```python
from build123d import *

# Parameters (mm, degrees)
SKETCH1_R                    = 77.5
SKETCH1_R_2                  = 56
BOSS_EXTRUDE1_DEPTH          = 5
SKETCH2_R                    = 2.75
CUT_EXTRUDE2_DEPTH           = 110.715541287
CHAMFER1_SIZE                = 0.5
CIRPATTERN1_COUNT            = 6
CHAMFER1_OF_CIRPATTERN1_SIZE = 0.5
CHAMFER2_SIZE                = 1


with BuildPart() as part:
    # Sketch1 → Boss-Extrude1 (new body)
    with BuildSketch(Plane(origin=(0, 0, 0), x_dir=(1, 0, 0), z_dir=(0, 1, 0))):
        with Locations(Location((0, 0, 0), (0, 0, 270))):
            Circle(SKETCH1_R)
        with Locations(Location((0, 0, 0), (0, 0, 270))):
            Circle(SKETCH1_R_2, mode=Mode.SUBTRACT)
    extrude(amount=BOSS_EXTRUDE1_DEPTH)

    # Sketch2 → Cut-Extrude2 (cut, through all)
    with BuildSketch(Plane(origin=(0, 5, 0), x_dir=(1, 0, 0), z_dir=(0, 1, 0))):
        with Locations(Location((0, 70.25, 0), (0, 0, 270))):
            Circle(SKETCH2_R)
    cut_extrude2 = extrude(amount=-CUT_EXTRUDE2_DEPTH, mode=Mode.SUBTRACT)

    # Chamfer1
    chamfer1_edges = [part.edges().sort_by_distance(p)[0] for p in [
        (0, 0, -73),
        (0, 5, -73),
    ]]
    chamfer(chamfer1_edges, length=CHAMFER1_SIZE)

    # CirPattern1: Cut-Extrude2 ×6 about axis
    cirpattern1_axis = Axis((0, 0, 0), (0, 1, 0))
    for i in range(1, CIRPATTERN1_COUNT):
        add(cut_extrude2.rotate(cirpattern1_axis, i * 360 / CIRPATTERN1_COUNT), mode=Mode.SUBTRACT)

    # Chamfer1 of CirPattern1
    chamfer1_of_cirpattern1_edges = [part.edges().sort_by_distance(p)[0] for p in [
        (-63.219854476, 0, -36.5),
        (-63.219854476, 5, -36.5),
        (-63.219854476, 0, 36.5),
        (-63.219854476, 5, 36.5),
        (0, 0, 73),
        (0, 5, 73),
        (63.219854476, 0, 36.5),
        (63.219854476, 5, 36.5),
        (63.219854476, 0, -36.5),
        (63.219854476, 5, -36.5),
    ]]
    chamfer(chamfer1_of_cirpattern1_edges, length=CHAMFER1_OF_CIRPATTERN1_SIZE)

    # Chamfer2
    chamfer2_edges = [part.edges().sort_by_distance(p)[0] for p in [
        (0, 5, -77.5),
        (0, 0, -56),
        (0, 5, -56),
    ]]
    chamfer(chamfer2_edges, length=CHAMFER2_SIZE)


solid = part.part
```
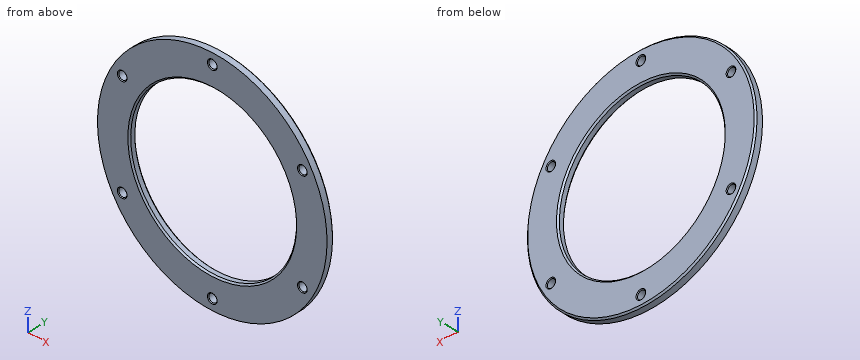
Here's how the part is built. I have some questions about the finished solid (model axes, mm). Give positions to 0.01 mm unless a question says otherwise; leave off trailing zeros. Order: outer loops, then holes, each group sorted by start corner. A loop starts at its lowest first (then second) coordinate and runs counter-clockwise, first axis right, second up. Notation, with made-up numbers: M -24,62.25 L 23,62.25 A25 ccw 23,87.25 Z; hole C 72.25,-19 d1. An arc over 180 degrees is marked long. Use a Markdown table: item, result. Add a question column.
1. Suppose I cut it at A-A (x = 0). Give the number of separate pieces and of enclosed holes in the cut face, and give its area (3 significant figures).
2. Suppose I cut it at C-C (y = 2.05). List the corners of the cut face in (x, z) for me (3 decimals).
3. Suppose I cut it at B-B (z = 0). List the corners of the cut face in (x, y) for me, and give its area (3 significant figures).
4. For pin 1 Ø5 at (x, z) = (-60.84, -35.13) entering from -Y; pin 2 Ø1 at (x, y) = (13.5, 3) entering from -Z; pin 3 Ø3 at (x, y) = (53.5, 2) entering from -Z; pin 4 Ø3 at (y, z) = (1, -44.5) entering from -X, each with a flat end and sliding along its axis, tell me the tip position at first contact or that it passes through.
5. I need wall thicknesses on probe 1 along X at (y, z) = (2.65, 0); probe 2 along Z at (x, y) = (46, 1.2); probe 3 along Z at (x, y) = (-15.5, 3.6). Which ranges of each line are inside material? Lowest first, please. Write a range as from..to.
Results list:
| question | item | result |
|---|---|---|
| 1 | separate pieces | 4 |
| 1 | enclosed holes | 0 |
| 1 | area | 156 mm² |
| 2 | outline | C 0,0 d155; hole C -60.838,-35.125 d5.5; hole C -60.838,35.125 d5.5; hole C 0,0 d112; hole C 0,-70.25 d5.5; hole C 0,70.25 d5.5; hole C 60.838,-35.125 d5.5; hole C 60.838,35.125 d5.5 |
| 3 | outline | M -77.5,0 L -57,0 L -56,1 L -56,4 L -57,5 L -76.5,5 L -77.5,4 Z; M 56,1 L 57,0 L 77.5,0 L 77.5,4 L 76.5,5 L 57,5 L 56,4 Z |
| 3 | area | 212 mm² |
| 4 | pin 1 | passes through |
| 4 | pin 2 | stops at z = -76.4 |
| 4 | pin 3 | stops at z = -57.47 |
| 4 | pin 4 | stops at x = -64.48 |
| 5 | probe 1 | x = -77.5..-56, 56..77.5 |
| 5 | probe 2 | z = -62.37..-31.94, 31.94..62.37 |
| 5 | probe 3 | z = -75.93..-53.81, 53.81..75.93 |
